Could you check a few things on this model? Use its own coordinates, in mm. Face numbers are marked on the shaded views. Round coordinates to 2 decimals unless told otherwise and drop trailing zeros. Loops run counter-clockwise (first coordinate to the right, second up) from the corner with the lowest first, then second, coordinate; pieces in that order, holes last. Notation, with made-up numbers: M 75.25,46.25 L 85.25,46.25 A26 cw 85.25,75.25 Z; hole C -21,-39.5 d8. An arc over 180 degrees is marked long. Answer in a Markdown table with one row per item.
```python
from build123d import *

# Parameters (mm, degrees)
SKETCH1_R           = 10.31875
SKETCH1_R_2         = 3.175
BOSS_EXTRUDE1_DEPTH = 4.7625
SKETCH6_R           = 1.3890625
CUT_EXTRUDE1_DEPTH  = 16.350394437


with BuildPart() as part:
    # Sketch1 → Boss-Extrude1 (new body)
    with BuildSketch(Plane.XY):
        with Locations(Location((0, 0, 0), (0, 0, 180))):
            Circle(SKETCH1_R)
        with Locations(Location((0, 0, 0), (0, 0, 180))):
            Circle(SKETCH1_R_2, mode=Mode.SUBTRACT)
    extrude(amount=BOSS_EXTRUDE1_DEPTH)

    # Sketch6 → Cut-Extrude1 (cut, through all)
    with BuildSketch(Plane.XY.offset(4.7625)):
        with Locations((0, 5.55625)):
            Circle(SKETCH6_R)
        with Locations((5.55625, 0)):
            Circle(SKETCH6_R)
        with Locations((0, -5.55625)):
            Circle(SKETCH6_R)
        with Locations((-5.55625, 0)):
            Circle(SKETCH6_R)
    extrude(amount=-CUT_EXTRUDE1_DEPTH, mode=Mode.SUBTRACT)


solid = part.part
```
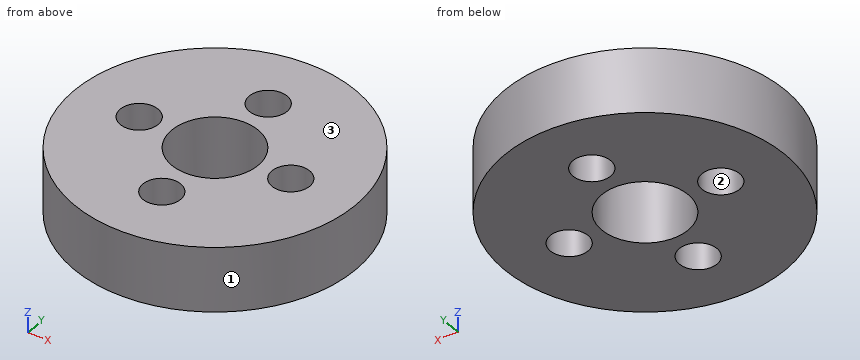
1) I want a section at A-A, the plane y = 0. Please give me the cut outline in (x, z) (1 decimal), plus the area to 3 significant figures.
Computed:
| item | result |
|---|---|
| outline | M -10.3,0 L -6.9,0 L -6.9,4.8 L -10.3,4.8 Z; M -4.2,0 L -3.2,0 L -3.2,4.8 L -4.2,4.8 Z; M 3.2,0 L 4.2,0 L 4.2,4.8 L 3.2,4.8 Z; M 6.9,0 L 10.3,0 L 10.3,4.8 L 6.9,4.8 Z |
| area | 41.6 mm² |
2) If we mould it in two halves opening along Y, with no side actions, what happens to the marked faces 1, 2 and 3? For each: released by +Y, released by -Y, zero draft, split by the parting line, or undercut.
Computed:
| item | result |
|---|---|
| face 1 | split by the parting line |
| face 2 | undercut |
| face 3 | zero draft |
3) I want a section at D-D, the plane z = 2. State how many separate pieces and enclosed holes the cut face has, plus the area to 3 significant figures.
Computed:
| item | result |
|---|---|
| separate pieces | 1 |
| enclosed holes | 5 |
| area | 279 mm² |
4) I need wall thicknesses on line 1 (Y direction, x = 0, z = 1.6) (3 decimals); line 2 (Y direction, x = -0.5, z = 1.55). Which ranges of each line are inside material? Lowest first, please.
Computed:
| item | result |
|---|---|
| line 1 | y = -10.319 to -6.945, -4.167 to -3.175, 3.175 to 4.167, 6.945 to 10.319 |
| line 2 | y = -10.31 to -6.85, -4.26 to -3.14, 3.14 to 4.26, 6.85 to 10.31 |
5) Will these pins go through, and if not, where does the flat tip stop? P1, Ø1, axis at y = 4.5, z = 1.5, coming from the +X side; P2, Ø1, axis at x = 1, z = 1.5, coming from the -Y side; P3, Ø1.5, axis at y = 6, z = 1, coming from the -X side.
Computed:
| item | result |
|---|---|
| P1 | stops at x = 9.51 |
| P2 | stops at y = -10.31 |
| P3 | stops at x = -8.88 |
6) I want a section at C-C, the plane x = 4.75. Please give me the cut outline in (y, z), plus the area to 3 significant figures.
Computed:
| item | result |
|---|---|
| outline | M -9.16,0 L -1.13,0 L -1.13,4.76 L -9.16,4.76 Z; M 1.13,0 L 9.16,0 L 9.16,4.76 L 1.13,4.76 Z |
| area | 76.5 mm² |
